Geometry: final body of the model. Coordinates: model frame, mm. A direction names the side the tool comes from. Coordinates: 2 decimals unless noted, no trailing zeros. Loops run counter-clockwise (first coordinate to the right, second up) from the corner with the lowest first, then second, coordinate; pieces in that order, holes last. Notation, with made-up numbers: (38.5, 56) -> (53.5, 56) arc R30 cw to (53.5, 78) -> close; hole circle Ø9 at (59, 76.25). An arc over 180 degrees is marked (long way). One line per item, written item: value. Start each with the question number.
Item 1: Section query D-D on z = -12. Return loops of the section in (x, y), then the cut area to 3 significant figures.
Item 2: Mould query, pull axis Y, two halves, no side actions, for faces 4 (the flat face through (-1, 0, 0)), 5 (the flat face through (-35, 3, -10)), 6 (the flat face through (-1, 6.88, 0)). Classes: +Y half, -Y half, draft (parallel to the pull), parting line (faces both ways), or undercut.
Item 3: Contact query for flat-ended pins moving along their axis: pin 1 Ø2 at (x, y) = (-4.5, 4) entering from +Z; pin 2 Ø2 at (y, z) = (5, -2) entering from -X; pin 3 Ø4 at (y, z) = (1, -3.5) entering from +X. Output: stop coordinate, or through.
Item 4: Section query C-C on y = 1.25. Return loops of the section in (x, z), then the cut area to 3 significant figures.
Item 5: Section query B-B on x = 25. Return loops of the section in (y, z).
Item 6: Set-up query: faces 1 (the flat face through (25, 3, -10)), 2 (the flat face through (5, 3, 10)), 3 (the flat face through (40, 3, 10)). Return all of +Z, -Z, +X, -X, +Y, -Y with unobstructed straight access to the full face (end or side cutting, diameter ignored); none if empty.
Item 7: Section query A-A on z = 0. Return loops of the section in (x, y).
Item 8: Ray query, probe 1 along X at (y, z) = (4.5, 0); probe 2 along X at (y, z) = (4.5, 10.25); probe 3 along X at (y, z) = (4.5, 12.25). Return the intervals inside material, ascending. Write a range as from..to.
from build123d import *

# Parameters (mm, degrees)
CROQUIS1_R              = 3.2
CROQUIS1_R_2            = 5
SALIENTE_EXTRUIR2_DEPTH = 6.88
SALIENTE_EXTRUIR3_DEPTH = 6.88
MATRIZL1_COUNT          = 2
MATRIZL1_PITCH          = 40
SIMETR_A1_COPY_1_DEPTH  = 6.88


with BuildPart() as part:
    # Croquis1 → Saliente-Extruir2 (new body)
    with BuildSketch(Plane(origin=(0, 0, 0), x_dir=(1, 0, 0), z_dir=(0, 1, 0))):
        with BuildLine():
            Line((-50, -10), (50, -10))
            ThreePointArc((50, -10), (60, 0), (50, 10))
            Line((50, 10), (-50, 10))
            ThreePointArc((-50, 10), (-60, 0), (-50, -10))
        make_face()
        with Locations(Location((-50, 0, 0), (0, 0, 270))):
            Circle(CROQUIS1_R, mode=Mode.SUBTRACT)
        with Locations(Location((50, 0, 0), (0, 0, 270))):
            Circle(CROQUIS1_R_2, mode=Mode.SUBTRACT)
    extrude(amount=SALIENTE_EXTRUIR2_DEPTH)

    # Croquis3 → Saliente-Extruir3 (add)
    with BuildSketch(Plane(origin=(0, 0, 0), x_dir=(1, 0, 0), z_dir=(0, 1, 0))):
        with BuildLine():
            Line((-20, -10), (-18, -10))
            ThreePointArc((-18, -10), (-15, -13), (-12, -10))
            Line((-12, -10), (-10, -10))
            ThreePointArc((-10, -10), (-15, -15), (-20, -10))
        make_face()
    saliente_extruir3 = extrude(amount=SALIENTE_EXTRUIR3_DEPTH)

    # MatrizL1: Saliente-Extruir3 ×2
    with Locations(*[(i * MATRIZL1_PITCH, 0, 0) for i in range(1, MATRIZL1_COUNT)]):
        add(saliente_extruir3)

    # Simetría1: Saliente-Extruir3 across plane
    add(saliente_extruir3.mirror(Plane.XY))

    # Simetría1 copy 1 sketch → Simetría1 copy 1 (add)
    with BuildSketch(Plane(origin=(40, 0, 0), x_dir=(1, 0, 0), z_dir=(0, 1, 0))):
        with BuildLine():
            Line((-20, 10), (-18, 10))
            ThreePointArc((-18, 10), (-15, 13), (-12, 10))
            Line((-12, 10), (-10, 10))
            ThreePointArc((-10, 10), (-15, 15), (-20, 10))
        make_face()
    extrude(amount=SIMETR_A1_COPY_1_DEPTH)


solid = part.part
Reply:
1. outline: (-19.58, 0) -> (-17.24, 0) -> (-17.24, 6.88) -> (-19.58, 6.88) -> close; (-12.76, 0) -> (-10.42, 0) -> (-10.42, 6.88) -> (-12.76, 6.88) -> close; (20.42, 0) -> (22.76, 0) -> (22.76, 6.88) -> (20.42, 6.88) -> close; (27.24, 0) -> (29.58, 0) -> (29.58, 6.88) -> (27.24, 6.88) -> close
1. area: 64.6 mm²
2. face 4: -Y half
2. face 5: draft
2. face 6: +Y half
3. pin 1: stops at z = 10
3. pin 2: stops at x = -59.95
3. pin 3: stops at x = 59.89
4. outline: (-50, -10) -> (-20, -10) arc R5 ccw to (-10, -10) -> (20, -10) arc R5 ccw to (30, -10) -> (50, -10) arc R10 ccw to (50, 10) -> (30, 10) arc R5 ccw to (20, 10) -> (-10, 10) arc R5 ccw to (-20, 10) -> (-50, 10) arc R10 ccw to start; hole circle Ø6.4 at (-50, 0); hole (-18, -10) arc R3 ccw to (-12, -10) -> close; hole (-18, 10) -> (-12, 10) arc R3 ccw to start; hole (22, -10) arc R3 ccw to (28, -10) -> close; hole (22, 10) -> (28, 10) arc R3 ccw to start; hole circle Ø10 at (50, 0)
4. area: 2,300 mm²
5. outline: (0, -15) -> (6.88, -15) -> (6.88, -13) -> (0, -13) -> close; (0, -10) -> (6.88, -10) -> (6.88, 10) -> (0, 10) -> close; (0, 13) -> (6.88, 13) -> (6.88, 15) -> (0, 15) -> close
6. face 1: +Y, -Y
6. face 2: +Z, +Y, -Y
6. face 3: +Z, +X, +Y, -Y
7. outline: (-60, 0) -> (-53.2, 0) -> (-53.2, 6.88) -> (-60, 6.88) -> close; (-46.8, 0) -> (45, 0) -> (45, 6.88) -> (-46.8, 6.88) -> close; (55, 0) -> (60, 0) -> (60, 6.88) -> (55, 6.88) -> close
8. probe 1: x = -60..-53.2, -46.8..45, 55..60
8. probe 2: x = -19.99..-17.99, -12.01..-10.01, 20.01..22.01, 27.99..29.99
8. probe 3: x = -19.47..-16.98, -13.02..-10.53, 20.53..23.02, 26.98..29.47
